Here's how the part is built. I have some questions about the finished solid (model axes, mm). A direction names the side the tool comes from. Coordinates: 2 decimals unless noted, no trailing zeros. Order: outer loops, then holes, each group sorted by start corner. A loop starts at its lowest first (then second) coordinate and runs counter-clockwise, first axis right, second up.
```python
from build123d import *

# Parameters (mm, degrees)
REVOLVE1_ANGLE          = 180
CUT_EXTRUDE1_REACH      = 114.566
CUT_EXTRUDE1_END_RADIUS = 31
SKETCH2_W               = 14
SKETCH2_H               = 8.185848791
SKETCH2_W_2             = 16
SKETCH2_H_2             = 15
CUT_EXTRUDE2_REACH      = 114.566
SKETCH3_R               = 1.525
CUT_EXTRUDE3_DEPTH      = 10
CUT_EXTRUDE4_REACH      = 128.25
SKETCH6_R               = 8.5


with BuildPart() as part:
    # Sketch1 → Revolve1 (revolve)
    with BuildSketch(Plane.XY):
        with BuildLine():
            Line((6.218316837, 14), (6.218316837, 6))
            Line((6.218316837, 6), (3.718316837, 6))
            Line((3.718316837, 6), (3.718316837, 24.731367941))
            Line((3.718316837, 24.731367941), (-10.171408573, 24.731367941))
            Line((-10.171408573, 24.731367941), (-27.781683163, 24.731367941))
            Line((-27.781683163, 24.731367941), (-27.781683163, 26.554502519))
            Line((-27.781683163, 26.554502519), (-35.281683163, 26.554502519))
            Line((-35.281683163, 26.554502519), (-35.281683163, 24.731367941))
            Line((-35.281683163, 24.731367941), (-38.281683163, 24.731367941))
            Line((-38.281683163, 24.731367941), (-38.281683163, 21.534346957))
            Line((-38.281683163, 21.534346957), (-59.281683163, 20.416426404))
            Line((-59.281683163, 20.416426404), (-59.281683163, 24.731367941))
            Line((-59.281683163, 24.731367941), (-59.281683163, 31))
            Line((-59.281683163, 31), (-56.981683163, 31))
            Line((-56.981683163, 31), (71.518316837, 31))
            add(Edge.make_bspline(
                [(71.518316837, 31), (87.336893309, 31), (105.518316837, 21.771712161), (105.518316837, 0)],
                knots=[0, 0, 0, 0, 1, 1, 1, 1], degree=3))
            Line((105.518316837, 0), (100.518316813, 0))
            add(Edge.make_bspline(
                [(71.518316837, 26), (84.501211561, 26), (100.518316813, 18.460024777), (100.518316813, 0)],
                knots=[0, 0, 0, 0, 1, 1, 1, 1], degree=3))
            Line((71.518316837, 26), (71.518316837, 14))
            Line((71.518316837, 14), (6.218316837, 14))
        make_face()
    revolve(axis=Axis((-52.937293729, 0, 0), (1, 0, 0)), revolution_arc=REVOLVE1_ANGLE)

    # Cut-Extrude1: up to this cylinder (the profile starts inside it)
    cut_extrude1_end = Plane(origin=(6.118317, 0, 0), z_dir=(-1, 0, 0)) * Cylinder(CUT_EXTRUDE1_END_RADIUS, 398.932, mode=Mode.PRIVATE)
    # Sketch2 → Cut-Extrude1 (cut, up to the surface)
    with BuildSketch(Plane(origin=(0, 0, 7), x_dir=(-1, 0, 0), z_dir=(0, 0, -1)), mode=Mode.PRIVATE) as cut_extrude1_sk1:
        with Locations((47.281683163, 26.907075605)):
            Rectangle(SKETCH2_W, SKETCH2_H)
    cut_extrude1_tool1 = extrude(cut_extrude1_sk1.sketch, amount=-CUT_EXTRUDE1_REACH, mode=Mode.PRIVATE) & cut_extrude1_end
    add(cut_extrude1_tool1.solids().sort_by_distance((-47.281683, 26.907076, 7))[0], mode=Mode.SUBTRACT)
    # Sketch2 → Cut-Extrude1 (cut, up to the surface)
    with BuildSketch(Plane(origin=(0, 0, 7), x_dir=(-1, 0, 0), z_dir=(0, 0, -1)), mode=Mode.PRIVATE) as cut_extrude1_sk2:
        with Locations((-59.518316837, -23.5)):
            Rectangle(SKETCH2_W_2, SKETCH2_H_2)
    cut_extrude1_tool2 = extrude(cut_extrude1_sk2.sketch, amount=-CUT_EXTRUDE1_REACH, mode=Mode.PRIVATE) & cut_extrude1_end
    add(cut_extrude1_tool2.solids().sort_by_distance((59.518317, -23.5, 7))[0], mode=Mode.SUBTRACT)
    # Sketch2 → Cut-Extrude1 (cut, up to the surface)
    with BuildSketch(Plane(origin=(0, 0, 7), x_dir=(-1, 0, 0), z_dir=(0, 0, -1)), mode=Mode.PRIVATE) as cut_extrude1_sk3:
        with Locations((-59.518316837, 23.5)):
            Rectangle(SKETCH2_W_2, SKETCH2_H_2)
    cut_extrude1_tool3 = extrude(cut_extrude1_sk3.sketch, amount=-CUT_EXTRUDE1_REACH, mode=Mode.PRIVATE) & cut_extrude1_end
    add(cut_extrude1_tool3.solids().sort_by_distance((59.518317, 23.5, 7))[0], mode=Mode.SUBTRACT)
    # Sketch2 → Cut-Extrude1 (cut, up to the surface)
    with BuildSketch(Plane(origin=(0, 0, 7), x_dir=(-1, 0, 0), z_dir=(0, 0, -1)), mode=Mode.PRIVATE) as cut_extrude1_sk4:
        with Locations((47.281683163, -26.907075605)):
            Rectangle(SKETCH2_W, SKETCH2_H)
    cut_extrude1_tool4 = extrude(cut_extrude1_sk4.sketch, amount=-CUT_EXTRUDE1_REACH, mode=Mode.PRIVATE) & cut_extrude1_end
    add(cut_extrude1_tool4.solids().sort_by_distance((-47.281683, -26.907076, 7))[0], mode=Mode.SUBTRACT)

    # Sketch3 → Cut-Extrude2 (cut, up to next)
    with BuildSketch(Plane.XY.offset(7), mode=Mode.PRIVATE) as cut_extrude2_sk1:
        with Locations((-47.281683163, 26.814151209)):
            Circle(SKETCH3_R)
    cut_extrude2_tool1 = extrude(cut_extrude2_sk1.sketch, amount=-CUT_EXTRUDE2_REACH, mode=Mode.PRIVATE) & part.part
    # Sketch3 → Cut-Extrude2 (cut, up to next)
    with BuildSketch(Plane.XY.offset(7), mode=Mode.PRIVATE) as cut_extrude2_sk2:
        with Locations(Location((-47.281683163, -26.814151209, 0), (0, 0, 90))):
            Circle(SKETCH3_R)
    cut_extrude2_tool2 = extrude(cut_extrude2_sk2.sketch, amount=-CUT_EXTRUDE2_REACH, mode=Mode.PRIVATE) & part.part
    # Sketch3 → Cut-Extrude2 (cut, up to next)
    with BuildSketch(Plane.XY.offset(7), mode=Mode.PRIVATE) as cut_extrude2_sk3:
        with Locations((59.518316837, 24)):
            Circle(SKETCH3_R)
    cut_extrude2_tool3 = extrude(cut_extrude2_sk3.sketch, amount=-CUT_EXTRUDE2_REACH, mode=Mode.PRIVATE) & part.part
    # Sketch3 → Cut-Extrude2 (cut, up to next)
    with BuildSketch(Plane.XY.offset(7), mode=Mode.PRIVATE) as cut_extrude2_sk4:
        with Locations((59.518316837, -24)):
            Circle(SKETCH3_R)
    cut_extrude2_tool4 = extrude(cut_extrude2_sk4.sketch, amount=-CUT_EXTRUDE2_REACH, mode=Mode.PRIVATE) & part.part
    add(cut_extrude2_tool1.solids().sort_by_distance((-47.281683, 26.814151, 7))[0], mode=Mode.SUBTRACT)
    add(cut_extrude2_tool2.solids().sort_by_distance((-47.281683, -26.814151, 7))[0], mode=Mode.SUBTRACT)
    add(cut_extrude2_tool3.solids().sort_by_distance((59.518317, 24, 7))[0], mode=Mode.SUBTRACT)
    add(cut_extrude2_tool4.solids().sort_by_distance((59.518317, -24, 7))[0], mode=Mode.SUBTRACT)

    # Sketch5 → Cut-Extrude3 (cut)
    with BuildSketch(Plane(origin=(0, 31, 0), x_dir=(1, 0, 0), z_dir=(0, 1, 0))):
        Polygon((4.441941487, 0), (11.658819852, -12.5), (26.092576582, -12.5), (33.309454947, 0), (26.092576582, 12.5), (11.658819852, 12.5), align=None)
    extrude(amount=-CUT_EXTRUDE3_DEPTH, mode=Mode.SUBTRACT)

    # Sketch6 → Cut-Extrude4 (cut, up to next)
    with BuildSketch(Plane(origin=(0, 31, 0), x_dir=(1, 0, 0), z_dir=(0, 1, 0)), mode=Mode.PRIVATE) as cut_extrude4_sk1:
        with Locations((81.518316837, 0)):
            Circle(SKETCH6_R)
    cut_extrude4_tool1 = extrude(cut_extrude4_sk1.sketch, amount=-CUT_EXTRUDE4_REACH, mode=Mode.PRIVATE) & part.part
    add(cut_extrude4_tool1.solids().sort_by_distance((81.518317, 31, 0))[0], mode=Mode.SUBTRACT)


solid = part.part
```
Q1. We'd pull the mould along X, two halves only. Please class faces 6 (the flat face through (51.518, -22, 14)), 7 (the flat face through (-59.282, 0, 23)): pulls with the +X half, pulls with the -X half, needs draft (parallel to the pull), parting line crosses it, or undercut.
Q2. Will these pins go through, and if not, where does the flat tip stop? pin 1 (3.5 mm diameter, centred on x = -44, y = -27, fed in from +Z); pin 2 (4 mm diameter, centred on x = -50.5, z = 15, fed in from +Y); pin 3 (8 mm diameter, centred on y = 0.5, z = 9, fed in from +X).
Q3. If we section it at B-B on z = 3: Give the number of separate pieces and of enclosed holes in the cut face, then the cut area to 3 significant figures.
Q4. For faces 1 (the flat face through (-40.282, -26, 12)), 2 (the flat face through (19, 25, 12.5)), 3 (the cylindrical face through (-48.794, -27.013, 3.549)), 4 (the conical face through (-48.929, 0.461, 20.962)), 5 (the flat face through (-40.282, 26, 12)), which set-ups out of +Z, -Z, +X, -X, +Y, -Y let a thin tool reach every point of the face, with its end or its side?
Q5. I need wall thicknesses on L1, parallel to X at y = 27.5, z = 3.5; L2, parallel to X at y = -23, z = 3.5; L3, parallel to X at y = 15, z = 17. Which ranges of each line are inside material? Lowest first, please.
Q6. If we section it at A-A on x = 54: Write out the boundary of the cut face in (y, z).
Q7. If we section it at D-D on x = -31.5: Write out the boundary of the cut face in (y, z).
Reply:
1. face 6: undercut
1. face 7: pulls with the -X half
2. pin 1: stops at z = 7
2. pin 2: stops at y = 22.81
2. pin 3: stops at x = 105.18
3. separate pieces: 2
3. enclosed holes: 4
3. area: 3,420 mm2
4. face 1: +Z, -Y
4. face 2: -Z, +Y
4. face 3: +Z, -Z
4. face 4: -Z
4. face 5: +Z, +Y
5. L1: x = -59.28 to -48.64, -45.92 to 6.46, 31.29 to 73.77
5. L2: x = -59.28 to -38.28, 3.72 to 58.37, 60.67 to 71.52, 85.04 to 94.96
5. L3: x = -59.28 to -38.28, 3.72 to 71.52, 86.34 to 95.67
6. outline: (-31, 0) - (-14, 0) arc R14 cw to (14, 0) - (31, 0) arc R31 ccw to (30.2, 7) - (16, 7) - (16, 26.55) arc R31 ccw to (-16, 26.55) - (-16, 7) - (-30.2, 7) arc R31 ccw to start
7. outline: (-31, 0) - (-26.55, 0) arc R26.55 cw to (26.55, 0) - (31, 0) arc R31 ccw to start
